The listing builds one solid part. Answer for the finished solid, in the listing's coordinates (mm). Face numbers are marked on the shaded views. Coordinates: 2 decimals unless noted, no trailing zeros. Write each loop counter-clockwise with the first axis right and the second up, starting at its lowest first coordinate (ties: lowest second). Pieces come first, ordered by that corner, then holes. Notation, with made-up numbers: M -3.75,-8.5 L 1.25,-8.5 A33 cw 1.25,19.5 Z; hole C -34,79.5 d2. An arc over 180 degrees is marked long. Write item = value, one per line. Start each with the question number.
Autodesk Inventor part; units mm, degrees
ref_plane "YZ Plane" through (0, 0, 0) normal (1, 0, 0) x (0, 1, 0)
ref_plane "XZ Plane" through (0, 0, 0) normal (0, 1, 0) x (-1, 0, 0)
ref_plane "XY Plane" through (0, 0, 0) normal (0, 0, 1) x (1, 0, 0)
sketch "Эскиз1" plane through (0, 0, 0) normal (0, 1, 0) x (-1, 0, 0)
  line L0 (-15.75, 7) -> (15.75, 7) construction
  line L1 (15.75, 7) -> (15.75, -7) construction
  line L2 (15.75, -7) -> (-15.75, -7) construction
  line L3 (-15.75, -7) -> (-15.75, 7) construction
  line L4 (-15.75, 7) -> (15.75, -7) construction
  line L5 (15.75, 7) -> (-15.75, -7) construction
  line L6 (0, 7) -> (-15.75, 7)
  line L7 (-15.75, 7) -> (-15.75, -7)
  line L8 (-15.75, -7) -> (0, -7)
  line L9 (0, -7) -> (0, 7)
  circle A0 centre (-8.75, 0) radius 1.6
  point P0 (0, 0)
  dimension "d0" = 31.5
  dimension "d1" = 14
  dimension "d2" = 3.2
  dimension "d3" = 7
extrude "Выдавливание1" add sketch "Эскиз1" along normal blind 2
sketch "Эскиз2" plane through (0, 2, 0) normal (0, 1, 0) x (1, 0, 0)
  circle A0 centre (8.75, 0) radius 1.6
  circle A1 centre (7.875, 9) radius 1.6
  circle A2 centre (7.875, -9) radius 1.6
  line L0 (0, -7) -> (15.75, -7)
  line L1 (15.75, 7) -> (0, 7)
  circle A3 centre (7.875, -9) radius 3
  circle A4 centre (7.875, 9) radius 3
  line L2 (0, 7) -> (6.1151, 11.4296)
  line L3 (9.6349, 11.4296) -> (15.75, 7)
  line L4 (15.75, -7) -> (15.75, 7)
  line L5 (0, 7) -> (0, -7)
  line L6 (0, -7) -> (6.1151, -11.4296)
  line L7 (15.75, -7) -> (9.6349, -11.4296)
  line L8 (7.875, 9) -> (7.875, -16.4074) construction
  point P0 (0, 0)
  point P1 (5.8526, -11.2158)
  point P2 (8.7863, -11.8582)
  point P3 (10.1111, -7)
  point P4 (5.6389, -7)
  dimension "d6" = 3.2
  dimension "d7" = 3.2
  dimension "d9" = 2
  dimension "d10" = 6
  dimension "d11" = 6
  dimension "d14" = 2
extrude "Выдавливание2" add sketch "Эскиз2" against normal blind 2 contours L0 A3 L6 | A3 L0 | L0 A3 | L2 A4 L1 | L0 L7 A3 | A4 L1 | A4 L3 L1 picked at (7.8107, 7.1372)
sketch "Эскиз3" plane through (0, 2, 0) normal (0, 1, 0) x (1, 0, 0)
  line L0 (2.75, -6) -> (4.75, -6)
  line L1 (4.75, -6) -> (4.75, 6)
  line L2 (4.75, 6) -> (2.75, 6)
  line L3 (2.75, 6) -> (2.75, -6)
  line L4 (2.75, -6) -> (4.75, 6) construction
  line L5 (4.75, -6) -> (2.75, 6) construction
  circle A0 centre (8.75, 0) radius 1.6
  point P0 (0, 0)
  point P1 (3.75, 0)
  dimension "d15" = 2
  dimension "d16" = 12
  dimension "d17" = 5
extrude "Выдавливание4" cut sketch "Эскиз3" against normal blind 2 contours L3 L2 L1 L0
properties part number "креп_отп_каретка"
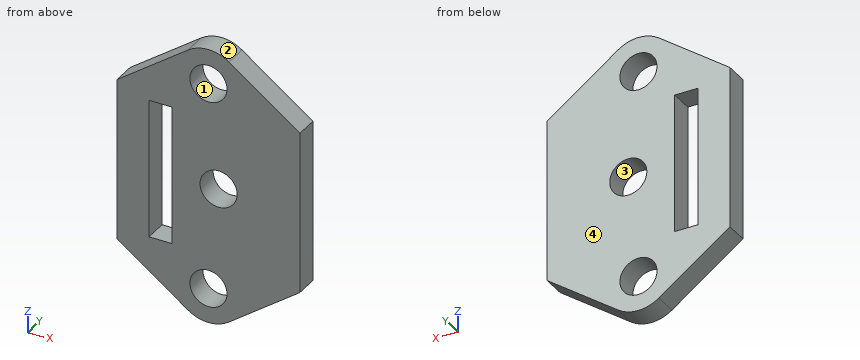
1. Straight lines are drawn through the part: L1, parallel to Z at x = 9, y = 0.6; L2, parallel to X at y = 0.7, z = -3.75; L3, parallel to Z at x = 8.5, y = 0.85. For each, find the intervals that lie inside material, in ascending order. Write a range as [from, to].
2. The part is cut by section C-C, the plane y = 1.25. Write down the section's boundary in (x, z) (3 decimals), and give its area (3 significant figures).
3. The part is cut by section D-D, the plane z = -9. Write down the section's boundary in (x, y) (3 decimals).
4. For a pull along Z with two mould halves and no side action, classify the marked faces 1, 2, 3 and 4 as pulls with the +Z half, pulls with the -Z half, needs draft (parallel to the pull), parting line crosses it, or undercut.
5. The part is cut by section A-A, the plane z = 2. Write down the section's boundary in (x, y), and give its area (3 significant figures).
6. The part is cut by section B-B, the plane x = 8.75. Write down the section's boundary in (y, z), and give its area (3 significant figures).
Solution:
q1.L1 = [-11.78, -10.14], [-7.86, -1.58], [1.58, 7.86], [10.14, 11.78]
q1.L2 = [0, 2.75], [4.75, 15.75]
q1.L3 = [-11.93, -10.47], [-7.53, -1.58], [1.58, 7.53], [10.47, 11.93]
q2.outline = M 0,-7 L 6.115,-11.43 A3 ccw 9.635,-11.43 L 15.75,-7 L 15.75,7 L 9.635,11.43 A3 ccw 6.115,11.43 L 0,7 Z; hole M 2.75,-6 L 4.75,-6 L 4.75,6 L 2.75,6 Z; hole C 7.875,-9 d3.2; hole C 7.875,9 d3.2; hole C 8.75,0 d3.2
q2.area = 260 mm^2
q3.outline = M 2.761,0 L 6.275,0 L 6.275,2 L 2.761,2 Z; M 9.475,0 L 12.989,0 L 12.989,2 L 9.475,2 Z
q4.face_1 = undercut
q4.face_2 = pulls with the +Z half
q4.face_3 = undercut
q4.face_4 = needs draft
q5.outline = M 0,0 L 2.75,0 L 2.75,2 L 0,2 Z; M 4.75,0 L 15.75,0 L 15.75,2 L 4.75,2 Z
q5.area = 27.5 mm^2
q6.outline = M 0,-11.87 L 2,-11.87 L 2,-10.34 L 0,-10.34 Z; M 0,-7.66 L 2,-7.66 L 2,-1.6 L 0,-1.6 Z; M 0,1.6 L 2,1.6 L 2,7.66 L 0,7.66 Z; M 0,10.34 L 2,10.34 L 2,11.87 L 0,11.87 Z
q6.area = 30.4 mm^2
